Autodesk Inventor part; units mm, degrees
ref_plane "YZ Plane" through (0, 0, 0) normal (1, 0, 0) x (0, 1, 0)
ref_plane "XZ Plane" through (0, 0, 0) normal (0, 1, 0) x (-1, 0, 0)
ref_plane "XY Plane" through (0, 0, 0) normal (0, 0, 1) x (1, 0, 0)
sketch "Sketch1" plane through (0, 0, 0) normal (0, 0, 1) x (1, 0, 0)
  line L0 (-4.25, 4.25) -> (4.25, 4.25)
  line L1 (4.25, 4.25) -> (4.25, -4.25)
  line L2 (4.25, -4.25) -> (-4.25, -4.25)
  line L3 (-4.25, -4.25) -> (-4.25, 4.25)
  point P0 (0, 0)
  dimension "d0" = 8.5
  dimension "d1" = 8.5
  dimension "d2" = 4.25
  dimension "d3" = 4.25
extrude "Extrusion1" add sketch "Sketch1" along normal blind 2.5
fillet "Fillet2" radius 1 3 edges at (4.25, 4.25, 1.25) (4.25, 0, 0) (0, 4.25, 0)
sketch "Sketch10" plane through (0, 0, 2.5) normal (0, 0, 1) x (1, 0, 0)
  line L0 (4.25, 3.25) -> (4.25, -4.25)
  line L1 (-4.25, 4.25) -> (3.25, 4.25)
  line L2 (3.25, 3.25) -> (-17.75, 3.25)
  line L3 (-17.75, 3.25) -> (-17.75, -17.75)
  line L4 (-17.75, -17.75) -> (3.25, -17.75)
  line L5 (3.25, -17.75) -> (3.25, 3.25)
  point P0 (0, 0)
  dimension "d113" = 1
  dimension "d114" = 1
  dimension "d115" = 21
  dimension "d116" = 21
extrude "Extrusion8" add sketch "Sketch10" along normal blind 7
hole "Hole9" at (3.25, -7.75, 6.5) direction (-1, 0, 0) diameter 2.3876 depth 5 tip angle 118 countersink diameter 2.54 countersink angle 120
hole "Hole10" at (-7.75, 3.25, 6.5) direction (0, -1, 0) diameter 2.3876 depth 5 tip angle 118 countersink diameter 2.54 countersink angle 120
hole "Hole11" at (-6.25, -6.25, 9.5) direction (0, 0, -1) diameter 6.35 depth 5
sketch "Sketch11" plane through (0, 0, 2.5) normal (0, 0, -1) x (-1, 0, 0)
  line L0 (17.75, -17.75) -> (-3.25, -17.75)
  line L1 (17.75, 3.25) -> (17.75, -17.75)
  line L2 (4.25, 3.25) -> (17.75, 3.25)
  line L3 (10.75, 3.25) -> (17.75, 3.25)
  line L4 (17.75, 3.25) -> (17.75, -17.75)
  line L5 (17.75, -17.75) -> (-3.25, -17.75)
  line L6 (-3.25, -17.75) -> (-3.25, -10.75)
  line L7 (-3.25, -10.75) -> (0.75, -10.75)
  line L8 (0.75, -10.75) -> (10.75, -0.75)
  line L9 (10.75, -0.75) -> (10.75, 3.25)
  point P0 (0, 0)
  dimension "d146" = 14
  dimension "d158" = 4
extrude "Extrusion9" cut sketch "Sketch11" against normal blind 3.325
hole "Hole12" at (-0.25, -14.75, 5.825) direction (0, 0, 1) diameter 2.3876 end through all countersink diameter 2.54 countersink angle 120
hole "Hole13" at (-14.75, -0.25, 5.825) direction (0, 0, 1) diameter 2.3876 end through all countersink diameter 2.54 countersink angle 120
chamfer "Chamfer3" distance 16 angle 45 1 edges at (-17.75, -17.75, 7.6625)
chamfer "Chamfer4" distance 1 angle 45 2 edges at (-7.25, 3.25, 9.5) (3.25, -7.25, 9.5)
sketch "Sketch15" plane through (0, 0, 2.5) normal (0, 0, 1) x (1, 0, 0)
  line L0 (-4.25, 3.25) -> (3.25, 3.25)
  line L1 (3.25, 3.25) -> (3.25, -4.25)
  line L2 (4.25, -4.25) -> (3.25, -4.25)
  line L3 (4.25, 3.25) -> (4.25, -4.25)
  arc A0 (4.25, 3.25) -> (3.25, 4.25) centre (3.25, 3.25) ccw
  line L4 (-4.25, 4.25) -> (3.25, 4.25)
  line L5 (-4.25, 3.25) -> (-4.25, 4.25)
  point P0 (0, 0)
extrude "Extrusion11" [suppressed]
chamfer "Chamfer6" distance 1 angle 45 1 edges at (3.25, 3.25, 5.5)
hole "Hole16" at (-0.5, -0.5, 0) direction (0, 0, 1) diameter 2.6924 end through all countersink diameter 3.302 countersink angle 120
sketch "Sketch16" plane through (0, 0, 2.5) normal (0, 0, -1) x (-1, 0, 0)
  line L0 (-3.25, -10.75) -> (0.75, -10.75)
  line L1 (10.75, -0.75) -> (10.75, 3.25)
  line L2 (4.25, 3.25) -> (10.75, 3.25)
  line L3 (4.25, -4.25) -> (4.25, 3.25)
  line L4 (-3.25, -4.25) -> (4.25, -4.25)
  line L5 (-3.25, -10.75) -> (-3.25, -4.25)
  line L6 (4.25, 4.25) -> (10.75, 4.25)
  line L7 (10.75, 4.25) -> (10.75, -0.75)
  line L8 (10.75, -0.75) -> (0.75, -10.75)
  line L9 (0.75, -10.75) -> (-4.25, -10.75)
  line L10 (-4.25, -10.75) -> (-4.25, -4.25)
  line L11 (-4.25, -4.25) -> (4.25, -4.25)
  line L12 (4.25, -4.25) -> (4.25, 4.25)
  point P0 (0, 0)
  dimension "d213" = 1
  dimension "d214" = 1
extrude "Extrusion12" add sketch "Sketch16" along normal blind 1
sketch "Sketch17" plane through (0, 0, 9.5) normal (0, 0, 1) x (1, 0, 0)
  circle A0 centre (-0.5, -0.5) radius 1.3462
  arc A1 (5.6176, -1.1176) -> (-1.1176, 5.6176) centre (2.25, 2.25) ccw
  line L0 (-3.8676, 2.8676) -> (-1.1176, 5.6176)
  line L1 (2.8676, -3.8676) -> (5.6176, -1.1176)
  arc A2 (-3.8676, 2.8676) -> (2.8676, -3.8676) centre (-0.5, -0.5) ccw
  line L2 (3.4997, 3.4997) -> (-5.0832, -5.0832) construction
  line L3 (3.25, -17.75) -> (3.25, 2.25)
  point P0 (0, 0)
  dimension "d221" = 9.525
  dimension "d222" = 3.75
extrude "Extrusion13" cut sketch "Sketch17" against normal blind 2.6
sketch "Sketch18" plane through (-17.75, 3.25, 5.825) normal (0, 1, 0) x (1, 0, 0)
  line L0 (21, -3.675) -> (13, -3.675)
  line L1 (13, -3.675) -> (13, 1.725)
  line L2 (14.6, 3.325) -> (21, 3.325)
  line L3 (21, 3.325) -> (21, -3.675)
  arc A0 (14.6, 3.325) -> (13, 1.725) centre (14.6, 1.725) ccw
  line L4 (21, -1.075) -> (21, 3.325)
  line L5 (20, -3.675) -> (16, -3.675)
  line L6 (7, 3.325) -> (21, 3.325)
  point P0 (17.75, 5.825)
  dimension "d223" = 1.6
  dimension "d224" = 8
extrude "Extrusion14" cut sketch "Sketch18" against normal blind 1
chamfer "Chamfer7" distance 1 angle 45 1 edges at (3.25, 2.25, 4.7)
properties part number "nub_minusZ_3_plunger" material "Aluminum-6061"
Check sheet for the modelled part. Datum: model origin and axes. Units: mm. A direction names the side the tool comes from. Round coordinates to 2 decimals unless told otherwise and drop trailing zeros. Order: outer loops, then holes, each group sorted by start corner. A loop starts at its lowest first (then second) coordinate and runs counter-clockwise, first axis right, second up.
1) Section check C-C (y = -12). Record the boundary of the cut face in (x, z) (3 decimals), and give its area (3 significant figures).
2) Section check B-B (z = 3.75). Record the boundary of the cut face in (x, y).
3) Scan lines: line 1 (Y direction, x = 1.5, z = 6.5); line 2 (Z direction, x = 2.1, y = -7.75); line 3 (Y direction, x = -0.5, z = 3). Record each from-to range of solid material in increasing order.
4) Section check A-A (x = -5.75). Record the boundary of the cut face in (y, z) (3 decimals).
5) Tool access check on faces 4 (the flat face through (-10.75, 1, 4)), 5 (the cylindrical face through (-8.76, 0.69, 7.14)), 6 (the flat face through (2.7, 1.8, 4.7)), 7 (the cylindrical face through (-3.15, -5.56, 6.96)). Record the directions out of +Z, -Z, +X, -X, +Y, -Y that give a thin tool (end or side, any length) a straight path to the whole face; none if there is none.
6) Go/stop test with flat-tipped pins: pin 1 Ø6 at (x, y) = (-4, -3.5) entering from +Z; pin 2 Ø1.5 at (x, y) = (-9, -10) entering from -Z (3 decimals); pin 3 Ø2.5 at (x, y) = (0.5, -2) entering from +Z; pin 4 Ø3 at (y, z) = (-11, 5.5) entering from -X. Record where each tip stops, or that it passes through.
7) Mould release check, pull along Y, two halves, no side actions. Record for faces 1 (the flat face through (4.25, -4, 2)), 2 (the flat face through (-5.7, -5.8, 3.2)), 3 (the cylindrical face through (-3.64, -4.08, 8.22)): +Y half, -Y half, draft (parallel to the pull), parting line (faces both ways), or undercut.
Result:
1. outline: (-7.5, 5.825) - (3.25, 5.825) - (3.25, 8.5) - (2.25, 9.5) - (-7.5, 9.5) - close
1. area: 39.0 mm2
2. outline: (-10.75, -0.75) - (-0.75, -10.75) - (3.25, -10.75) - (3.25, 1.25) - (2.25, 2.25) - (-4.71, 2.25) - (-4.71, 3.25) - (-10.75, 3.25) - close; hole circle Ø2.69 at (-0.5, -0.5)
3. line 1: y = -17.75 to -8.94, -6.56 to 2.25
3. line 2: z = 1.5 to 5.31, 7.69 to 9.5
3. line 3: y = -10.75 to -1.85, 0.85 to 2.25
4. outline: (-13.75, 5.825) - (-9.385, 5.825) - (-9.385, 9.5) - (-13.75, 9.5) - close; (-5.75, 1.5) - (4.25, 1.5) - (4.25, 2.5) - (3.25, 2.5) - (3.25, 8.5) - (2.25, 9.5) - (-3.115, 9.5) - (-3.115, 4.5) - (-5.75, 4.5) - close
5. face 4: -Z, -X, +Y, -Y
5. face 5: +Y
5. face 6: +Z, +X, +Y
5. face 7: +Z
6. pin 1: stops at z = 9.5
6. pin 2: stops at z = 5.825
6. pin 3: stops at z = 6.9
6. pin 4: stops at x = -9.96
7. face 1: draft
7. face 2: -Y half
7. face 3: undercut
